Design review of the part built by this model. Coordinates are the model's own, in mm. Face numbers are marked on the shaded views. A direction names the side the tool comes from. Give positions to 0.01 mm unless a question says otherwise; leave off trailing zeros. Order: outer loops, then holes, each group sorted by start corner. A loop starts at its lowest first (then second) coordinate and runs counter-clockwise, first axis right, second up.
Autodesk Inventor part; units mm, degrees
ref_plane "YZ Plane" through (0, 0, 0) normal (1, 0, 0) x (0, 1, 0)
ref_plane "XZ Plane" through (0, 0, 0) normal (0, 1, 0) x (-1, 0, 0)
ref_plane "XY Plane" through (0, 0, 0) normal (0, 0, 1) x (1, 0, 0)
sketch "Sketch1" plane through (0, 0, 0) normal (0, 1, 0) x (-1, 0, 0)
  line L0 (0, 0) -> (28, 0)
  line L1 (28, 0) -> (28, -38.5)
  line L2 (28, -38.5) -> (0, -38.5)
  line L3 (0, -38.5) -> (0, 0)
  dimension "d0" = 28
  dimension "d1" = 38.5
extrude "Extrusion1" add sketch "Sketch1" along normal blind 3
sketch "Sketch2" plane through (0, 3, 0) normal (0, 1, 0) x (1, 0, 0)
  line L0 (-28, 0) -> (0, 0)
  circle A0 centre (0, 0) radius 2
  circle A1 centre (-28, 0) radius 2
  line L1 (0, 38.5) -> (-28, 38.5)
  circle A2 centre (-28, 38.5) radius 2
  circle A3 centre (0, 38.5) radius 2
  dimension "d8" = 4
  dimension "d9" = 4
  dimension "d10" = 4
  dimension "d11" = 4
extrude "Extrusion2" cut sketch "Sketch2" against normal blind 3
sketch "Sketch3" plane through (0, 3, 0) normal (0, 1, 0) x (1, 0, 0)
  line L0 (-32.85, 43.35) -> (4.85, 43.35)
  line L1 (4.85, 43.35) -> (4.85, -4.85)
  line L2 (4.85, -4.85) -> (-32.85, -4.85)
  line L3 (-32.85, -4.85) -> (-32.85, 43.35)
  line L4 (-2, 38.5) -> (-26, 38.5)
  line L5 (0, 2) -> (0, 36.5)
  point P0 (0, 0)
  point P1 (-2, 6.25)
  point P2 (-26, 32.25)
  dimension "d14" = 48.2
  dimension "d15" = 37.7
  dimension "d16" = 4.85
  dimension "d17" = 4.85
extrude "Extrusion3" add sketch "Sketch3" along normal blind 2
sketch "Sketch4" plane through (0, 3, 0) normal (0, -1, 0) x (1, 0, 0)
  circle A0 centre (2.35, -40.85) radius 2.25
  line L0 (-2, -38.5) -> (-26, -38.5)
  line L1 (0, -2) -> (0, -36.5)
  circle A1 centre (-30.35, -40.85) radius 2.25
  line L2 (-28, -36.5) -> (-28, -2)
  circle A2 centre (-30.35, 2.35) radius 2.25
  line L3 (-26, 0) -> (-2, 0)
  circle A3 centre (2.35, 2.35) radius 2.25
  point P0 (0, 0)
  dimension "d20" = 4.5
  dimension "d21" = 2.35
  dimension "d22" = 2.35
  dimension "d23" = 4.5
  dimension "d24" = 2.35
  dimension "d25" = 2.35
  dimension "d26" = 4.5
  dimension "d27" = 2.35
  dimension "d28" = 4.5
  dimension "d29" = 2.35
  dimension "d30" = 2.35
  dimension "d31" = 2.35
extrude "Extrusion4" add sketch "Sketch4" along normal blind 3
fillet "Fillet1" radius 2 4 edges at (4.85, 4, -43.35) (4.85, 4, 4.85) (-32.85, 4, 4.85) (-32.85, 4, -43.35)
sketch "Sketch5" plane through (0, 5, 0) normal (0, 1, 0) x (1, 0, 0)
  circle A0 centre (0, 19.25) radius 1
  circle A1 centre (-28, 19.25) radius 1
  line L0 (4.85, -2.85) -> (4.85, 41.35)
  line L1 (-30.85, -4.85) -> (2.85, -4.85)
  point P0 (0, 0)
  dimension "d45" = 2
  dimension "d46" = 2
  dimension "d73" = 28
  dimension "d81" = 24.1
  dimension "d82" = 4.85
extrude "Extrusion6" cut sketch "Sketch5" against normal through all
sketch "Sketch8" plane through (0, 5, 0) normal (0, 1, 0) x (1, 0, 0)
  circle A0 centre (-14, 3.125) radius 1.75
  line L0 (-2, 6.25) -> (-26, 6.25)
  line L1 (-26, 0) -> (-2, 0)
  line L2 (-32.85, 41.35) -> (-32.85, -2.85)
  point P0 (0, 0)
  dimension "d68" = 3.5
  dimension "d69" = 3.125
  dimension "d70" = 18.85
extrude "Extrusion9" cut sketch "Sketch8" against normal through all
sketch "Sketch9" plane through (0, 5, 0) normal (0, 1, 0) x (1, 0, 0)
  circle A0 centre (-14, 3.125) radius 1.75
  line L0 (-15, 4.5611) -> (-15, 6.25)
  line L1 (-15, 6.25) -> (-13, 6.25)
  line L2 (-13, 6.25) -> (-13, 4.5611)
  arc A1 (-13, 4.5611) -> (-15, 4.5611) centre (-14, 3.125) ccw
  line L3 (-2, 6.25) -> (-26, 6.25)
  point P0 (0, 0)
  point P1 (-14, 6.25)
  dimension "d76" = 2
  dimension "d77" = 1
extrude "Extrusion10" cut sketch "Sketch9" against normal through all contours A0 L0 L1 L2
fillet "Fillet2" radius 2 2 edges at (-15, 2.5, -4.5611) (-13, 2.5, -4.5611)
sketch "Sketch10" plane through (0, 5, 0) normal (0, 1, 0) x (1, 0, 0)
  line L0 (-25.5, 12.75) -> (-2.5, 12.75)
  line L1 (-2.5, 12.75) -> (-2.5, 25.75)
  line L2 (-2.5, 25.75) -> (-25.5, 25.75)
  line L3 (-25.5, 25.75) -> (-25.5, 12.75)
  line L4 (-32.85, 41.35) -> (-32.85, -2.85)
  circle A0 centre (-28, 19.25) radius 1
  point P0 (0, 0)
  dimension "d83" = 23
  dimension "d84" = 13
  dimension "d85" = 7.35
  dimension "d86" = 6.5
extrude "Extrusion11" cut sketch "Sketch10" against normal through all contours L3 L2 L1 L0
sketch "Sketch11" plane through (0, 5, 0) normal (0, 1, 0) x (1, 0, 0)
  line L0 (4.85, -4.85) -> (-32.85, -4.85)
  line L1 (-32.85, -4.85) -> (-32.85, 12.75)
  line L2 (-32.85, 12.75) -> (4.85, 12.75)
  line L3 (4.85, 12.75) -> (4.85, -4.85)
  line L4 (-2.5, 12.75) -> (-25.5, 12.75)
  point P0 (0, 0)
  point P1 (-32.85, -2.85)
  point P2 (2.85, -4.85)
  point P3 (4.85, -2.85)
extrude "Extrusion12" cut sketch "Sketch11" against normal through all
sketch "Sketch12" plane through (0, 5, 0) normal (0, 1, 0) x (1, 0, 0)
  circle A0 centre (-14, 35.375) radius 2.5
  line L0 (-2, 38.5) -> (-26, 38.5)
  line L1 (4.85, 12.75) -> (4.85, 41.35)
  point P0 (0, 0)
  point P1 (-14, 38.5)
  dimension "d92" = 5
  dimension "d93" = 3.125
  dimension "d94" = 18.85
extrude "Extrusion13" cut sketch "Sketch12" against normal through all
sketch "Sketch13" plane through (0, 5, 0) normal (0, 1, 0) x (1, 0, 0)
  circle A0 centre (-14, 35.375) radius 2.5
  line L0 (-15.5, 33.375) -> (-15.5, 25.75)
  line L1 (-2.5, 25.75) -> (-25.5, 25.75)
  line L2 (-12.5, 33.375) -> (-12.5, 19.264)
  point P0 (0, 0)
  point P1 (-12.5, 25.75)
  dimension "d97" = 3
extrude "Extrusion14" cut sketch "Sketch13" against normal through all contours A0 L2 L1 L0
fillet "Fillet3" radius 2 2 edges at (-12.5, 2.5, -33.375) (-15.5, 2.5, -33.375)
sketch "Sketch14" plane through (-30.35, 0, -40.85) normal (0, -1, 0) x (1, 0, 0)
  circle A0 centre (32.7, 0) radius 2.25
  circle A1 centre (0, 0) radius 2.25
  circle A2 centre (32.7, 0) radius 1.15
  circle A3 centre (0, 0) radius 1.15
  point P0 (30.35, 40.85)
  dimension "d101" = 2.3
  dimension "d102" = 2.3
extrude "Extrusion15" cut sketch "Sketch14" against normal through all contours A2 | A3
sketch "Sketch16" plane through (0, 5, 0) normal (0, 1, 0) x (1, 0, 0)
  line L0 (-25.5, 25.75) -> (-25.5, 12.75)
  line L1 (-32.85, 41.35) -> (-32.85, 12.75)
  line L2 (-25.5, 12.75) -> (-32.85, 12.75)
  line L3 (-32.85, 12.75) -> (-32.85, 16.75)
  line L4 (-32.85, 16.75) -> (-25.5, 16.75)
  line L5 (-25.5, 16.75) -> (-25.5, 12.75)
  line L6 (-2.5, 25.75) -> (-2.5, 12.75)
  line L7 (4.85, 12.75) -> (4.85, 41.35)
  line L8 (-2.5, 12.75) -> (4.85, 12.75)
  line L9 (4.85, 12.75) -> (4.85, 16.75)
  line L10 (4.85, 16.75) -> (-2.5, 16.75)
  line L11 (-2.5, 16.75) -> (-2.5, 12.75)
  point P0 (0, 0)
  point P1 (1.175, 12.75)
  point P2 (-2.5, 16.75)
  dimension "d109" = 4
  dimension "d110" = 4
extrude "Extrusion17" cut sketch "Sketch16" against normal blind 2
properties part number "ServoFullMountInsert"
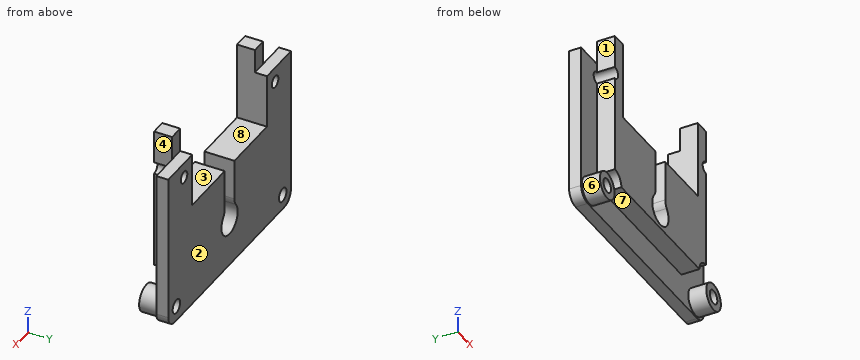
1. Take a section at B-B (x = 2.35). State the section outline as (y, z) points.
Recorded:
outline: (0, -43.1) - (3, -43.1) - (3, -43.35) - (5, -43.35) - (5, -42) - (0, -42) - close; (0, -39.7) - (5, -39.7) - (5, -16.75) - (3, -16.75) - (3, -38.6) - (0, -38.6) - close
2. Take a section at C-C (z = -24). State the section outline as (x, y) points, then the cut area to 3 significant figures.
Recorded:
outline: (-32.85, 3) - (-28, 3) - (-28, 0) - (-25.5, 0) - (-25.5, 5) - (-32.85, 5) - close; (-2.5, 0) - (0, 0) - (0, 3) - (4.85, 3) - (4.85, 5) - (-2.5, 5) - close
area: 44.4 mm2
3. For pin 1 (1 mm diameter, centred on x = 1.5, y = 4.5, fed in from +Z); pin 2 (1.5 mm diameter, centred on y = 2, z = -30, fed in from -X); pin 3 (1.5 mm diameter, centred on x = 0.5, z = -24, fed in from -Y); pin 4 (0.9 mm diameter, centred on y = 1.5, z = -14.5, fed in from +X), all flat-tipped, find the tip position at first contact; note any pin that passes through.
Recorded:
pin 1: stops at z = -16.75
pin 2: stops at x = -28
pin 3: stops at y = 0
pin 4: stops at x = 0
4. Take a section at D-D (y = 4.5). State the section outline as (x, z) points (3 decimals).
Recorded:
outline: (-32.85, -41.35) arc R2 ccw to (-30.85, -43.35) - (2.85, -43.35) arc R2 ccw to (4.85, -41.35) - (4.85, -16.75) - (-2.5, -16.75) - (-2.5, -25.75) - (-12.5, -25.75) - (-12.5, -32.547) arc R2 ccw to (-12.056, -33.804) arc R2.5 cw (long way) to (-15.944, -33.804) arc R2 ccw to (-15.5, -32.547) - (-15.5, -25.75) - (-25.5, -25.75) - (-25.5, -16.75) - (-32.85, -16.75) - close; hole circle Ø2.3 at (-30.35, -40.85); hole circle Ø2 at (-28, -19.25); hole circle Ø2 at (0, -19.25); hole circle Ø2.3 at (2.35, -40.85)
5. Take a section at A-A (z = -40.85). State the section outline as (x, y) points, then the cut area to 3 significant figures.
Recorded:
outline: (-32.85, 3) - (-32.6, 3) - (-32.6, 0) - (-31.5, 0) - (-31.5, 5) - (-32.85, 5) - close; (-29.2, 0) - (-28.1, 0) - (-28.1, 3) - (0.1, 3) - (0.1, 0) - (1.2, 0) - (1.2, 5) - (-29.2, 5) - close; (3.5, 0) - (4.6, 0) - (4.6, 3) - (4.85, 3) - (4.85, 5) - (3.5, 5) - close
area: 79.4 mm2
6. For line 1 along X through (y, z) = (3.8, -19.25); line 2 along Z through (x, y) = (-30.5, 2.55) (3 decimals); line 3 along X through (y, z) = (1, -31), list the stretches that pass through material, from the lowest coordinate up.
Recorded:
line 1: x = -32.85 to -29, -27 to -25.5, -2.5 to -1, 1 to 4.85
line 2: z = -43.095 to -41.99, -39.71 to -38.605
line 3: x = -28 to -15.5, -12.5 to 0
7. Draft analysis for pull direction X (two halves, no side actions). For the marked faces 1, 2 and 3, state which applies: pulls with the +X half, pulls with the -X half, needs draft (parallel to the pull), parting line crosses it, or undercut.
Recorded:
face 1: pulls with the -X half
face 2: needs draft
face 3: undercut
8. Machinability: for the marked faces 4, 5, 6, 7 and 8, which of the approach directions +Z, -Z, +X, -X, +Y, -Y give a long, thin tool a straight path to every point of the face, cutting with its end or side? Answer none if there is none.
Recorded:
face 4: +Z, -Z, +X, -Y
face 5: +Z, -Z, -X, -Y
face 6: -Y
face 7: -Z, +X, -X, -Y
face 8: +Z, +Y, -Y
